The drawing under review shows one solid part. Ordinate dimensions are in mm from its lowest x, y, z. A direction names the side the tool comes from. Coordinates: 2 decimals unless noted, no trailing zeros. Write each loop counter-clockwise with the first axis right and the second up, starting at its lowest first coordinate (ties: lowest second). Pieces come first, ordered by that corner, then holes.
Q1. To check wall thickness, follow probe 1 along Z at (x, y) = (18, 0.6); probe 2 along X at (y, z) = (1.8, 21.5) (1 decimal); probe 3 along Z at (x, y) = (31, 3.95) (1 decimal). State the ranges of each line that lie inside material, in increasing order.
Q2. Add section A-A, the plane z = 15. Give the boundary of the cut face in (x, y), plus the area to 3 significant figures.
Q3. The part is to be moulded in two halves that separate along Z. For the marked faces 1, 2 and 3, say which applies: +Z half, -Z half, draft (parallel to the pull), parting line (faces both ways), or undercut.
Q4. Machinability: for the marked faces 4, 5 and 6, which of the approach directions +Z, -Z, +X, -X, +Y, -Y give a long, thin tool a straight path to every point of the face, cutting with its end or side? Answer none if there is none.
Q5. Add section B-B, the plane x = 18.5. Give the boundary of the cut face in (y, z).
Q6. Add section C-C, the plane y = 0.8. Give the boundary of the cut face in (x, z).
Q7. Clearance check with flat-ended pins moving along their axes: pin 1 Ø3 at (x, y) = (25, 2.5) entering from +Z; pin 2 Ø2.5 at (x, y) = (1.5, 3) entering from +Z; pin 3 Ø2 at (x, z) = (9.5, 14) entering from -Y; pin 4 Ø1 at (y, z) = (4, 25.5) entering from -X. State where each tip first meets the part, or that it passes through.
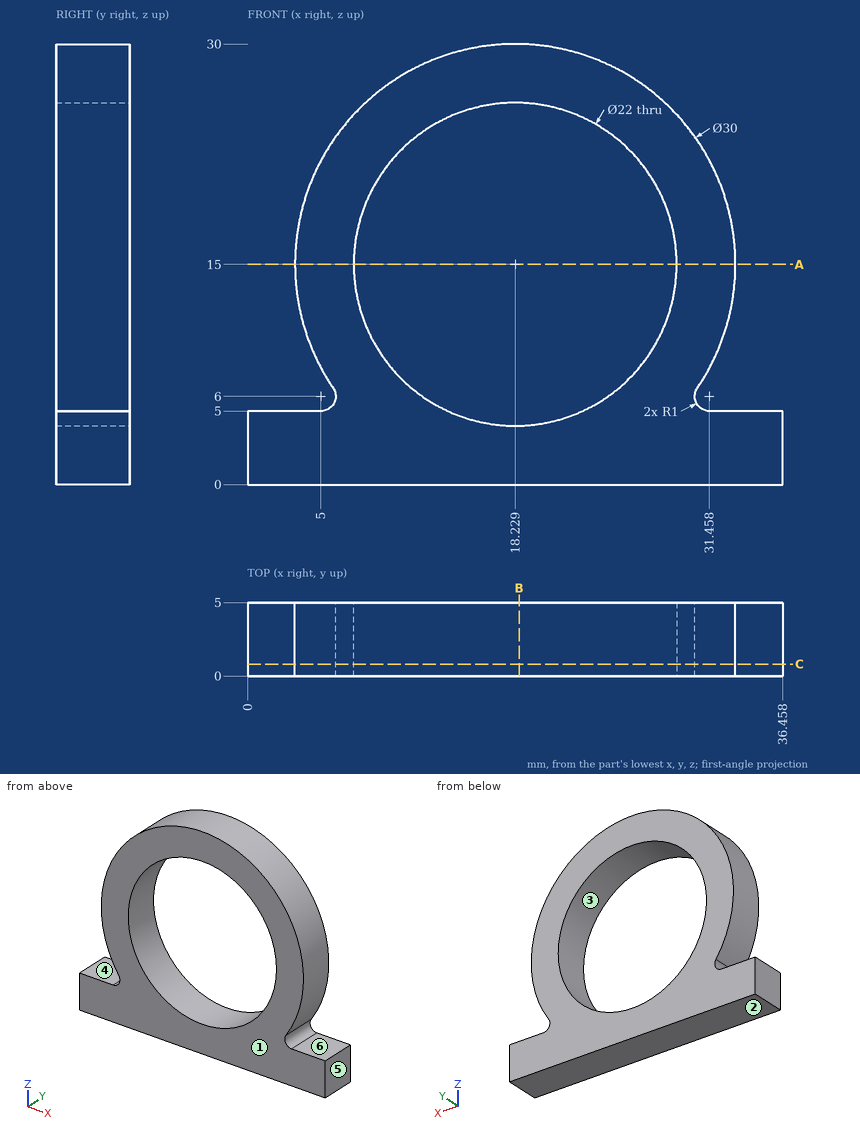
Here are the results:
1. probe 1: z = 0 to 4, 26 to 30
1. probe 2: x = 4.7 to 9.4, 27.1 to 31.7
1. probe 3: z = 0 to 5.1, 7.1 to 22.9
2. outline: (3.23, 0) - (7.23, 0) - (7.23, 5) - (3.23, 5) - close; (29.23, 0) - (33.23, 0) - (33.23, 5) - (29.23, 5) - close
2. area: 40.0 mm2
3. face 1: draft
3. face 2: -Z half
3. face 3: undercut
4. face 4: -X, +Y, -Y
4. face 5: +Z, -Z, +X, +Y, -Y
4. face 6: +X, +Y, -Y
5. outline: (0, 0) - (5, 0) - (5, 4) - (0, 4) - close; (0, 26) - (5, 26) - (5, 30) - (0, 30) - close
6. outline: (0, 0) - (36.46, 0) - (36.46, 5) - (31.46, 5) arc R1 cw to (30.63, 6.56) arc R15 ccw (long way) to (5.83, 6.56) arc R1 cw to (5, 5) - (0, 5) - close; hole circle Ø22 at (18.23, 15)
7. pin 1: stops at z = 29.04
7. pin 2: stops at z = 5
7. pin 3: passes through
7. pin 4: stops at x = 7.05
